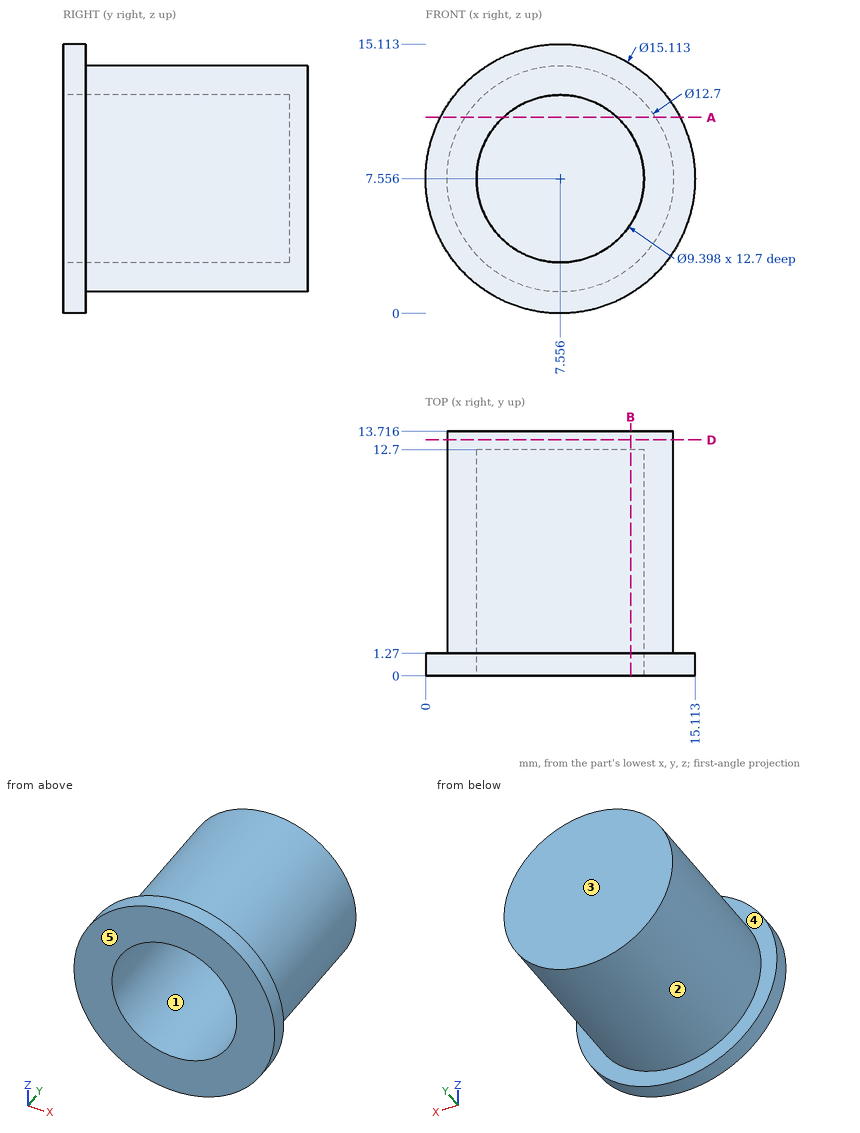
Verification items for this drawing (mm, ordinates from the low corner). A direction names the side the tool comes from. Give positions to 0.01 mm unless a question says otherwise; leave off trailing zeros. Write each loop counter-clockwise with the first axis right and the second up, starting at its lowest first coordinate (ties: lowest second). Pieces come first, ordered by that corner, then holes. Notation, with made-up numbers: (5.25, 88) - (20.25, 88) arc R34 cw to (20.25, 118) - close; hole circle Ø7 at (9, 58.25). An arc over 180 degrees is marked (long way). Answer as CSV lines item,"result". Start each with the question number.
1. Sectioned sample at D-D (y = 13.25). Record the boundary of the cut face in (x, z).
2. Sectioned sample at B-B (x = 11.5). Record the boundary of the cut face in (y, z) (1 decimal).
3. Thickness scan on line 1 (Y direction, x = 6.25, z = 5.25) (1 decimal); line 2 (Y direction, x = 1.25, z = 11); line 3 (X direction, y = 5.5, z = 9.25) (1 decimal). Record the ranges inside material, lowest first.
4. Draft check along X on the marked faces 1, 2 and 3. Enter one of: pulls with the +X half, pulls with the -X half, needs draft (parallel to the pull), parting line crosses it, or undercut.
5. Depth check by flat-ended pin: pin 1 (5 mm diameter, centred on y = 3, z = 5.5, fed in from -X); pin 2 (2 mm diameter, centred on x = 12, y = 7.5, fed in from -Z); pin 3 (5 mm diameter, centred on x = 6, y = 4, fed in from -Z). Enter the tip coordinate at first touch or a pass-through.
6. Set-up check for the marked faces 4 and 5: record each of +Z, -Z, +X, -X, +Y, -Y from which the full face is reachable in a straight line by a thin tool's end or side.
7. Sectioned sample at A-A (z = 11). Record the boundary of the cut face in (x, y) (1 decimal).
Derived:
1,outline,"circle Ø12.7 at (7.56, 7.56)"
2,outline,"(0, 1.1) - (1.3, 1.1) - (1.3, 2.6) - (13.7, 2.6) - (13.7, 12.5) - (1.3, 12.5) - (1.3, 14) - (0, 14) - (0, 10.1) - (12.7, 10.1) - (12.7, 5) - (0, 5) - close"
3,line 1,"12.7 to 13.7"
3,line 2,"0 to 1.27"
3,line 3,"1.4 to 3.2, 11.9 to 13.7"
4,face 1,"undercut"
4,face 2,"parting line crosses it"
4,face 3,"needs draft"
5,pin 1,"x = 0"
5,pin 2,"z = 2.22"
5,pin 3,"z = 1.21"
6,face 4,"+Y"
6,face 5,"+Z, -Z, +X, -X, -Y"
7,outline,"(0.8, 0) - (4.4, 0) - (4.4, 12.7) - (10.8, 12.7) - (10.8, 0) - (14.3, 0) - (14.3, 1.3) - (12.9, 1.3) - (12.9, 13.7) - (2.2, 13.7) - (2.2, 1.3) - (0.8, 1.3) - close"
